Part model, mm, in its own coordinate system. A direction names the side the tool comes from. Round coordinates to 2 decimals unless told otherwise and drop trailing zeros. Write each loop counter-clockwise with the first axis right and the second up, starting at its lowest first coordinate (ties: lowest second). Pieces come first, ordered by that corner, then holes.
```python
from build123d import *

# Parameters (mm, degrees)
F2_R     = 1.27
F3_R     = 9.525
F4_DEPTH = 30.481


with BuildPart() as f1:
    # F0 (on Front) → F1 (revolve)
    with BuildSketch(Plane.XZ):
        Polygon((-14.656985, 26.67), (-14.656985, 0), (15.823015, 0), (15.823015, 26.67), (12.806601, 26.67), (12.806601, 24.527449), (11.443161, 24.527449), (11.443161, 26.67), (-10.664052, 26.67), (-10.664052, 25.014395), (-12.027493, 25.014395), (-12.027493, 26.67), align=None)
    revolve(axis=Axis((0.34086, 0, 0), (1, 0, 0)))

    # F2
    f2_edges = [f1.edges().sort_by_distance(p)[0] for p in [
        (-14.656985, 0, -26.67),
        (15.823015, 0, -26.67),
    ]]
    fillet(f2_edges, radius=F2_R)

    # F3 (on face) → F4 (cut, through all)
    with BuildSketch(Plane.YZ.offset(15.823015)):
        with Locations((10.10793, 7.688937)):
            Circle(F3_R)
    extrude(amount=-F4_DEPTH, mode=Mode.SUBTRACT)


solid = f1.part
```
Q1. Which spindle directions (+Z, -Z, +X, -X, +Y, -Y) get a long thin tool onto all of the face, cutting with end or side? Do faces 1 (the cylindrical face through (13.668, -26.443, -3.472)), 2 (the flat face through (11.443, 22, -12)). Say none if no direction does.
Values follow:
face 1: +X, -X
face 2: none
Q2. Drop flat-ended pins along their axis: pin 1 (3 mm diameter, centred on x = 10.5, z = 17.5, fed in from +Y); pin 2 (12 mm diameter, centred on x = -5, y = -12, fed in from +Z); pin 3 (6 mm diameter, centred on x = 1.5, y = -11.5, fed in from +Z); pin 4 (11.5 mm diameter, centred on y = 10.11, z = 7.69, fed in from +X). Give the stop position or say it passes through.
Values follow:
pin 1: stops at y = 21.34
pin 2: stops at z = 25.99
pin 3: stops at z = 25.28
pin 4: passes through
Q3. Mould opens along Y. For faces 3 (the flat face through (-14.657, 0, 0)), 4 (the cylindrical face through (0.8, 8, -1.6)), 5 (the cylindrical face through (12.115, -7.367, 23.395)) say: +Y half, -Y half, draft (parallel to the pull), parting line (faces both ways), or undercut.
Values follow:
face 3: draft
face 4: undercut
face 5: parting line
Q4. Cut at A-A on z = 0. Write the cut outline in (x, y), plus the area to 3 significant figures.
Values follow:
outline: (-14.66, -25.4) arc R1.27 ccw to (-13.39, -26.67) - (-12.03, -26.67) - (-12.03, -25.01) - (-10.66, -25.01) - (-10.66, -26.67) - (11.44, -26.67) - (11.44, -24.53) - (12.81, -24.53) - (12.81, -26.67) - (14.55, -26.67) arc R1.27 ccw to (15.82, -25.4) - (15.82, 4.49) - (-14.66, 4.49) - close; (-14.66, 15.73) - (15.82, 15.73) - (15.82, 25.4) arc R1.27 ccw to (14.55, 26.67) - (12.81, 26.67) - (12.81, 24.53) - (11.44, 24.53) - (11.44, 26.67) - (-10.66, 26.67) - (-10.66, 25.01) - (-12.03, 25.01) - (-12.03, 26.67) - (-13.39, 26.67) arc R1.27 ccw to (-14.66, 25.4) - close
area: 1,270 mm2
Q5. Cut at B-B on x = -4.5. Write the cut outline in (y, z) (3 decimals), plus the area to 3 significant figures.
Values follow:
outline: circle Ø53.34 at (0, 0); hole circle Ø19.05 at (10.108, 7.689)
area: 1,950 mm2
Q6. Wall check: L1, parallel to X at y = -15, z = -20.5; L2, parallel to Z at x = 14, y = 12; L3, parallel to Z at x = 12.5, y = 9.5. Give the ranges that are in metal, low to high.
Values follow:
L1: x = -14.66 to -12.03, -10.66 to 11.44, 12.81 to 15.82
L2: z = -23.82 to -1.65, 17.02 to 23.82
L3: z = -22.61 to -1.82, 17.19 to 22.61
